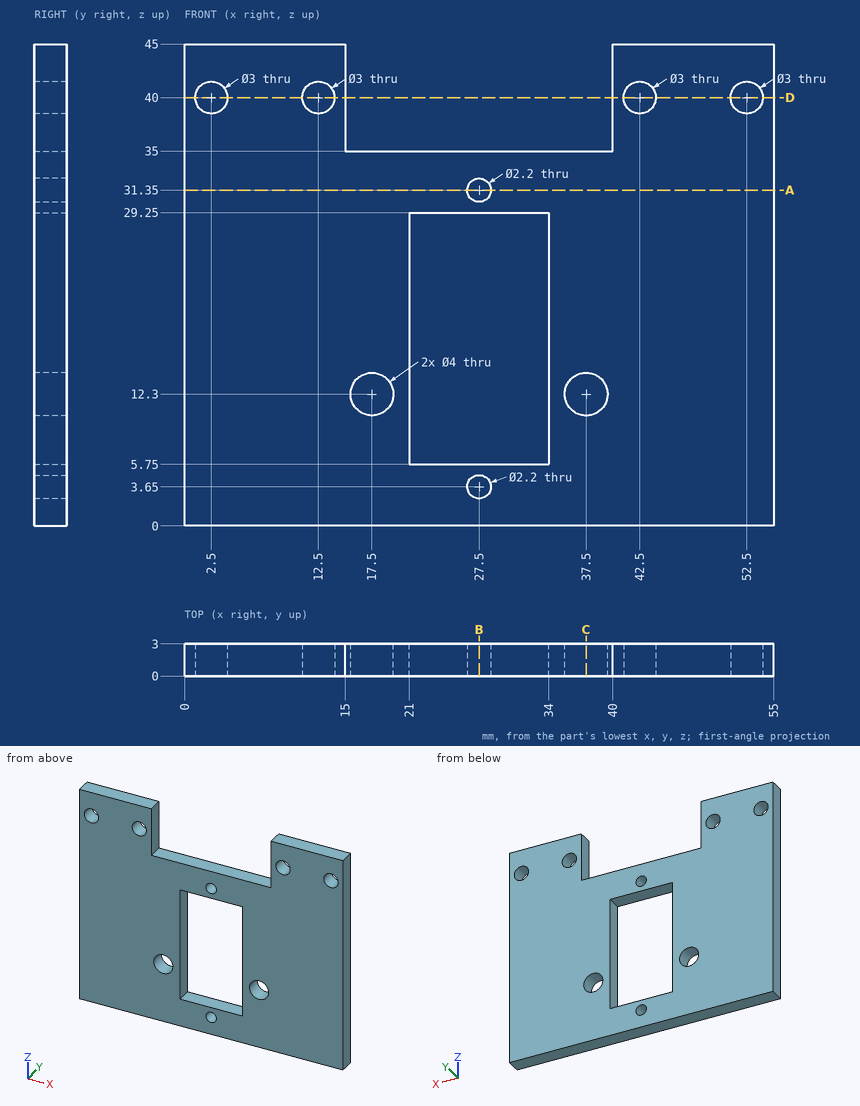
Study the drawing (mm; zero at the part's minimum x, y, z) and answer. Give positions to 0.01 mm unless a question says otherwise; leave off trailing zeros. Loops run counter-clockwise (first coordinate to the right, second up) from the corner with the lowest first, then second, coordinate; pieces in that order, holes last. Notation, with made-up numbers: M -26,86 L 21,86 A10 cw 21,93 Z; hole C 45.5,23 d10. An arc over 180 degrees is marked long. One line per item, written item: value. Start each with the question number.
1. This flat-tipped pin is pushed along its axis until it touches: P1, Ø0.9, axis at x = 29.5, y = 1, coming from the +Z side. Where does it stop, or does it pass through?
2. Find the intervals of material crossed by probe 1 along X at (y, z) = (0.7, 40); probe 2 along X at (y, z) = (2, 21); probe 3 along Z at (x, y) = (52.5, 1.2), in increasing order.
3. Find section D-D (z = 40). Give the vertices of the cut face in (x, y).
4. Find section C-C (x = 37.5). Give the vertices of the cut face in (y, z).
5. Find section A-A (z = 31.35). Give the vertices of the cut face in (x, y).
6. Find section B-B (x = 27.5). Give the vertices of the cut face in (y, z), and give its area (3 significant figures).
Reported:
1. P1: stops at z = 35
2. probe 1: x = 0 to 1, 4 to 11, 14 to 15, 40 to 41, 44 to 51, 54 to 55
2. probe 2: x = 0 to 21, 34 to 55
2. probe 3: z = 0 to 38.5, 41.5 to 45
3. outline: M 0,0 L 1,0 L 1,3 L 0,3 Z; M 4,0 L 11,0 L 11,3 L 4,3 Z; M 14,0 L 15,0 L 15,3 L 14,3 Z; M 40,0 L 41,0 L 41,3 L 40,3 Z; M 44,0 L 51,0 L 51,3 L 44,3 Z; M 54,0 L 55,0 L 55,3 L 54,3 Z
4. outline: M 0,0 L 3,0 L 3,10.3 L 0,10.3 Z; M 0,14.3 L 3,14.3 L 3,35 L 0,35 Z
5. outline: M 0,0 L 26.4,0 L 26.4,3 L 0,3 Z; M 28.6,0 L 55,0 L 55,3 L 28.6,3 Z
6. outline: M 0,0 L 3,0 L 3,2.55 L 0,2.55 Z; M 0,4.75 L 3,4.75 L 3,5.75 L 0,5.75 Z; M 0,29.25 L 3,29.25 L 3,30.25 L 0,30.25 Z; M 0,32.45 L 3,32.45 L 3,35 L 0,35 Z
6. area: 21.3 mm²
